Model file for the job. Use its own axes, mm. Face numbers are marked on the shaded views. A direction names the side the tool comes from. Round coordinates to 2 decimals unless told otherwise and drop trailing zeros. Loops run counter-clockwise (first coordinate to the right, second up) from the corner with the lowest first, then second, coordinate; pieces in that order, holes last. Notation, with made-up numbers: (-11, -37.5) -> (31, -37.5) arc R31 ccw to (31, -13.5) -> close; hole circle Ø3 at (88.25, -2). An arc over 180 degrees is marked (long way). Use a Markdown table: item, result.
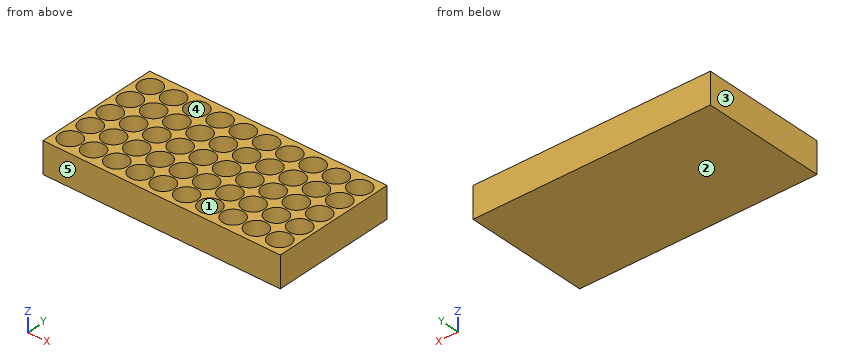
from build123d import *

# Parameters (mm, degrees)
CYLINDER_R     = 7
CYLINDER_DEPTH = 20
ARRAY_X_COUNT  = 10
ARRAY_X_PITCH  = 15
ARRAY_Y_COUNT  = 5
ARRAY_Y_PITCH  = 15
BOX_W          = 153
BOX_H          = 80
BOX_DEPTH      = 20


with BuildPart() as obj1:
    # Cylinder → Cylinder (new body)
    with BuildSketch(Plane.XY.offset(2)):
        Circle(CYLINDER_R)
    extrude(amount=CYLINDER_DEPTH)

    # Array X: obj1 ×10


with BuildPart() as obj1_1:
    add(obj1.part)
    with Locations(*[(i * ARRAY_X_PITCH, 0, 0) for i in range(1, ARRAY_X_COUNT)]):
        add(obj1.part)

    # Array Y: obj1 ×5


with BuildPart() as obj1_2:
    add(obj1_1.part)
    with Locations(*[(0, i * ARRAY_Y_PITCH, 0) for i in range(1, ARRAY_Y_COUNT)]):
        add(obj1_1.part)


with BuildPart() as obj2:
    # Box → Box (new body)
    with BuildSketch(Plane(origin=(-9, -10, 0), x_dir=(1, 0, 0), z_dir=(0, 0, 1))):
        with Locations((76.5, 40)):
            Rectangle(BOX_W, BOX_H)
    extrude(amount=BOX_DEPTH)

    # Cut: cut obj1
    add(obj1_2.part, mode=Mode.SUBTRACT)


solid = obj2.part
Q1. Flat gauge pin, fed straight in: pin 1 (4 mm diameter, centred on x = 2.5, y = 13.5, fed in from +Z). Where does the tip first touch, or does it go through?
Results list:
| item | result |
|---|---|
| pin 1 | stops at z = 2 |
Q2. Band-saw the part on B-B, the plane x = 60. Give the cut face in (y, z), plus the area to 3 significant figures.
Results list:
| item | result |
|---|---|
| outline | (-10, 0) -> (70, 0) -> (70, 20) -> (67, 20) -> (67, 2) -> (53, 2) -> (53, 20) -> (52, 20) -> (52, 2) -> (38, 2) -> (38, 20) -> (37, 20) -> (37, 2) -> (23, 2) -> (23, 20) -> (22, 20) -> (22, 2) -> (8, 2) -> (8, 20) -> (7, 20) -> (7, 2) -> (-7, 2) -> (-7, 20) -> (-10, 20) -> close |
| area | 340 mm² |
Q3. Band-saw the part on A-A, the plane z = 4.5. Give the number of separate pieces and of enclosed holes in the cut face, plus the area to 3 significant figures.
Results list:
| item | result |
|---|---|
| separate pieces | 1 |
| enclosed holes | 50 |
| area | 4,540 mm² |
Q4. Band-saw the part on C-C, the plane x = 17. Give the cut face in (y, z).
Results list:
| item | result |
|---|---|
| outline | (-10, 0) -> (70, 0) -> (70, 20) -> (66.71, 20) -> (66.71, 2) -> (53.29, 2) -> (53.29, 20) -> (51.71, 20) -> (51.71, 2) -> (38.29, 2) -> (38.29, 20) -> (36.71, 20) -> (36.71, 2) -> (23.29, 2) -> (23.29, 20) -> (21.71, 20) -> (21.71, 2) -> (8.29, 2) -> (8.29, 20) -> (6.71, 20) -> (6.71, 2) -> (-6.71, 2) -> (-6.71, 20) -> (-10, 20) -> close |
Q5. Drill centre lines: L1, parallel to Y at x = 60, z = 7; L2, parallel to Y at x = 26, z = 15; L3, parallel to Z at x = 49.5, y = 20. Where is each one in solid material? Low to high. Write a range as from..to.
Results list:
| item | result |
|---|---|
| L1 | y = -10..-7, 7..8, 22..23, 37..38, 52..53, 67..70 |
| L2 | y = -10..-5.74, 5.74..9.26, 20.74..24.26, 35.74..39.26, 50.74..54.26, 65.74..70 |
| L3 | z = 0..2 |
Q6. Tool access for the marked faces 4 and 5: list every direction of +Z, -Z, +X, -X, +Y, -Y with a clear straight run to the whole face (end or side of a thin tool).
Results list:
| item | result |
|---|---|
| face 4 | +Z |
| face 5 | +Z, -Z, +X, -X, -Y |
Q7. Pull direction X, two halves, no side cores. Call the marked faces 1, 2 and 3: released by +X, released by -X, zero draft, split by the parting line, or undercut.
Results list:
| item | result |
|---|---|
| face 1 | undercut |
| face 2 | zero draft |
| face 3 | released by -X |
